Verification items for the finished model (mm, model axes). A direction names the side the tool comes from. Round coordinates to 2 decimals unless told otherwise and drop trailing zeros. Order: outer loops, then holes, each group sorted by start corner. A loop starts at its lowest first (then second) coordinate and runs counter-clockwise, first axis right, second up.
Autodesk Inventor part; units mm, degrees
ref_plane "YZ Plane" through (0, 0, 0) normal (1, 0, 0) x (0, 1, 0)
ref_plane "XZ Plane" through (0, 0, 0) normal (0, 1, 0) x (-1, 0, 0)
ref_plane "XY Plane" through (0, 0, 0) normal (0, 0, 1) x (1, 0, 0)
sketch "Sketch1" plane through (0, 0, 0) normal (0, 1, 0) x (-1, 0, 0)
  circle A0 centre (0, 0) radius 59
  circle A1 centre (0, 0) radius 81
  circle A2 centre (0, 0) radius 87.5
  line L0 (90, -56) -> (15, -56)
  line L1 (10, -51) -> (10, 51)
  line L2 (15, 56) -> (90, 56)
  line L3 (90, 56) -> (90, -56)
  line L4 (90, -56) -> (10, 56) construction
  line L5 (10, -56) -> (90, 56) construction
  arc A3 (10, -51) -> (15, -56) centre (15, -51) ccw
  arc A4 (15, 56) -> (10, 51) centre (15, 51) ccw
  point P0 (50, 0)
  point P1 (90, 0)
  point P2 (10, 0)
  point P3 (60, -54.4151)
  point P4 (60, 54.4151)
  point P5 (80, 35.4436)
  point P6 (80, -35.4436)
  point P7 (67.2328, 56)
  point P8 (67.2328, -56)
  dimension "d0" = 118
  dimension "d1" = 162
  dimension "d2" = 175
  dimension "d7" = 112
  dimension "d9" = 80
  dimension "d10" = 10
  dimension "d11" = 5
extrude "Extrusion1" add sketch "Sketch1" along normal blind 5 contours A0 L0 A1 L2 | A1 L0 A2 L2 picked at (42.125, 58.7621) picked at (-85.0936, 2.0693)
fillet "Fillet1" radius 5 4 edges at (-67.2328, 2.5, -56) (-67.2328, 2.5, 56) (-18.5742, 2.5, -56) (-18.5742, 2.5, 56)
sketch "Sketch2" plane through (0, 5, 0) normal (0, 1, 0) x (1, 0, 0)
  circle A0 centre (0, 0) radius 70.375
  line L0 (-36.4414, 79.1184) -> (-50.2978, 71.1184)
  line L1 (-50.2978, 71.1184) -> (-44.9056, 61.7788)
  arc A1 (-31.0492, 69.7788) -> (-44.9056, 61.7788) centre (0, 0) ccw
  line L2 (-31.0492, 69.7788) -> (-36.4414, 79.1184)
  circle A2 centre (-40.5, 70.1481) radius 3.5625
  circle A3 centre (-40.5, 70.1481) radius 3.5625
  line L3 (86.7392, -8) -> (86.7392, 8)
  line L4 (86.7392, 8) -> (75.9549, 8)
  arc A4 (75.9549, -8) -> (75.9549, 8) centre (0, 0) ccw
  line L5 (75.9549, -8) -> (86.7392, -8)
  arc A5 (80.9215, -3.5651) -> (80.9217, -3.5616) centre (0, 0) ccw
  arc A6 (81.0783, -3.5616) -> (80.9217, -3.5616) centre (81, 0) ccw
  line L6 (81.0783, -3.5616) -> (80.9215, -3.5651)
  line L7 (-50.2978, -71.1184) -> (-36.4414, -79.1184)
  line L8 (-36.4414, -79.1184) -> (-31.0492, -69.7788)
  arc A7 (-44.9056, -61.7788) -> (-31.0492, -69.7788) centre (0, 0) ccw
  line L9 (-44.9056, -61.7788) -> (-50.2978, -71.1184)
  circle A8 centre (-40.5, -70.1481) radius 3.5625
  point P0 (-65.1143, 450.6181)
extrude "Extrusion2" cut sketch "Sketch2" against normal blind 10 contours A2 | A5 A6 L6 | A8
properties part number "Cylinder Segment Holder"
1) Sectioned sample at B-B on x = 0. Record the cut outline in (y, z), then the cut area to 3 significant figures.
2) Tool access check on faces 5 (the cylindrical face through (81.16, 2.54, -3.56)), 6 (the flat face through (-37, 2, 56)). Record the directions out of +Z, -Z, +X, -X, +Y, -Y that give a thin tool (end or side, any length) a straight path to the whole face; none if there is none.
3) Sectioned sample at D-D on z = 33. Record the cut outline in (x, y), then the cut area to 3 significant figures.
4) Scan lines: probe 1 along Z at (x, y) = (-2, 3.2); probe 2 along Z at (x, y) = (-40.5, 1.5); probe 3 along Z at (x, y) = (-16.5, 3.75). Record each from-to range of solid material in increasing order.
5) Draft check along Z on faces 1 (the cylindrical face through (87.454, 2.465, -2.829)), 2 (the cylindrical face through (-60.18, 2.54, 59.12)), 3 (the flat face through (64, 5, 1)), 4 (the cylindrical face through (-38.86, 2.54, 73.31)). Enter one of: released by +Z, released by -Z, zero draft, split by the parting line, or undercut.
6) Sectioned sample at C-C on y = 4.1. Count the separate pieces of the cut face and the enclosed holes in it, then the cut area to 3 significant figures.
7) Go/stop test with flat-tipped pins: pin 1 Ø2 at (y, z) = (1, 19.5) entering from +X; pin 2 Ø1 at (y, z) = (4, -21.5) entering from +X; pin 3 Ø4.5 at (x, z) = (-40.5, 70.15) entering from +Y; pin 4 Ø3 at (y, z) = (1, -44) entering from -X. Record where each tip stops, or that it passes through.
8) Sectioned sample at A-A on z = 0. Record the cut outline in (x, y), then the cut area to 3 significant figures.
Returned:
1. outline: (0, -87.5) - (5, -87.5) - (5, -59) - (0, -59) - close; (0, 59) - (5, 59) - (5, 87.5) - (0, 87.5) - close
1. area: 285 mm2
2. face 5: +Y, -Y
2. face 6: -X, +Y, -Y
3. outline: (48.91, 0) - (81.04, 0) - (81.04, 5) - (48.91, 5) - close
3. area: 161 mm2
4. probe 1: z = -87.48 to -58.97, 58.97 to 87.48
4. probe 2: z = -77.56 to -73.71, -66.59 to -56, 56 to 66.59, 73.71 to 77.56
4. probe 3: z = -85.93 to -56.65, 56.65 to 85.93
5. face 1: split by the parting line
5. face 2: undercut
5. face 3: zero draft
5. face 4: undercut
6. separate pieces: 1
6. enclosed holes: 3
6. area: 9,250 mm2
7. pin 1: stops at x = 85.52
7. pin 2: stops at x = 84.94
7. pin 3: passes through
7. pin 4: stops at x = 37.56
8. outline: (59, 0) - (77.44, 0) - (77.44, 5) - (59, 5) - close; (84.56, 0) - (87.5, 0) - (87.5, 5) - (84.56, 5) - close
8. area: 107 mm2
